from build123d import *

# Parameters (mm, degrees)
F0_W     = 30.0482
F0_H     = 30.0482
F1_DEPTH = 28.3972
F2_W     = 26.543
F2_H     = 26.543
F3_DEPTH = 27.1272
F4_R     = 0.508


with BuildPart() as f1:
    # F0 (on Front) → F1 (new body)
    with BuildSketch(Plane.XZ):
        with Locations((1.779277, -2.752393)):
            Rectangle(F0_W, F0_H)
    extrude(amount=F1_DEPTH)

    # F2 (on face) → F3 (cut)
    with BuildSketch(Plane.XZ.offset(28.3972)):
        with Locations((1.804677, -2.777793)):
            Rectangle(F2_W, F2_H)
    extrude(amount=-F3_DEPTH, mode=Mode.SUBTRACT)

    # F4
    f4_edges = [f1.edges().sort_by_distance(p)[0] for p in [
        (-13.244823, -14.1986, 12.271707),
        (-13.244823, -14.1986, -17.776493),
        (16.803377, -14.1986, 12.271707),
        (16.803377, -14.1986, -17.776493),
    ]]
    fillet(f4_edges, radius=F4_R)


solid = f1.part
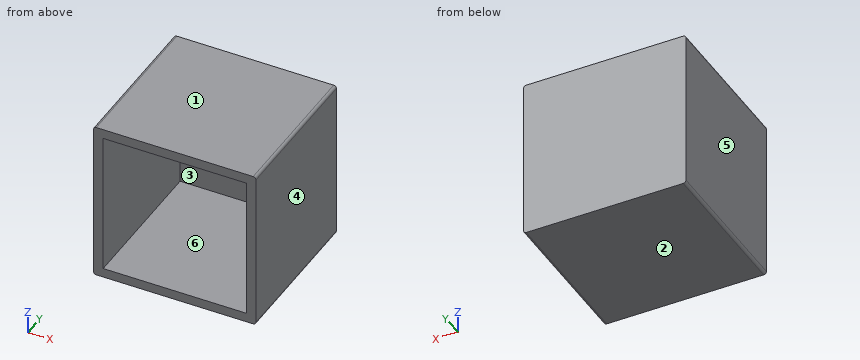
Read the model definition and answer for the solid it produces. Units are mm, in the model's axes. Face numbers are marked on the shaded views. A direction names the side the tool comes from. Coordinates: 2 decimals unless noted, no trailing zeros. Loops run counter-clockwise (first coordinate to the right, second up) from the corner with the lowest first, then second, coordinate; pieces in that order, holes last. Notation, with made-up numbers: (-9.5, 75.5) - (31.5, 75.5) arc R34 ccw to (31.5, 113.5) - close; hole circle Ø9 at (50, 8.25). An arc over 180 degrees is marked (long way). Answer in a Markdown table with one row per item.
Q1. For the marked faces 5 and 6, determine the directions among +Z, -Z, +X, -X, +Y, -Y from which every point of the face is accessible in a straight line to the end or side of a thin tool.
Here are the results:
| item | result |
|---|---|
| face 5 | +Z, -Z, -X, +Y, -Y |
| face 6 | -Y |
Q2. Find section C-C on z = 6.5. Write down the section's boundary in (x, y), plus the area to 3 significant figures.
Here are the results:
| item | result |
|---|---|
| outline | (-13.24, -28.4) - (-11.47, -28.4) - (-11.47, -1.27) - (15.08, -1.27) - (15.08, -28.4) - (16.8, -28.4) - (16.8, 0) - (-13.24, 0) - close |
| area | 133 mm^2 |
Q3. The mould has two halves that part along Z. Classify the marked faces 1, 2, 3 and 4: pulls with the +Z half, pulls with the -Z half, needs draft (parallel to the pull), parting line crosses it, or undercut.
Here are the results:
| item | result |
|---|---|
| face 1 | pulls with the +Z half |
| face 2 | pulls with the -Z half |
| face 3 | undercut |
| face 4 | needs draft |
Q4. Find section B-B on x = 2.5. Write down the section's boundary in (y, z).
Here are the results:
| item | result |
|---|---|
| outline | (-28.4, -17.78) - (0, -17.78) - (0, 12.27) - (-28.4, 12.27) - (-28.4, 10.49) - (-1.27, 10.49) - (-1.27, -16.05) - (-28.4, -16.05) - close |
Q5. Given P1, Ø1.5, axis at x = -8, z = -8.5, coming from the -Y side, flat-ended and moving along its own axis, determine where the tip first touches the part or whether it passes through.
Here are the results:
| item | result |
|---|---|
| P1 | stops at y = -1.27 |
Q6. Straight lines are drawn through the part: line 1 along X through (y, z) = (-10.5, -2.5); line 2 along Z through (x, y) = (-8.5, -24); line 3 along Y through (x, z) = (3, -9). For each, find the intervals that lie inside material, in ascending order. Write a range as [from, to].
Here are the results:
| item | result |
|---|---|
| line 1 | x = [-13.24, -11.47], [15.08, 16.8] |
| line 2 | z = [-17.78, -16.05], [10.49, 12.27] |
| line 3 | y = [-1.27, 0] |
Q7. Find section A-A on y = -2. Write down the section's boundary in (x, z), plus the area to 3 significant figures.
Here are the results:
| item | result |
|---|---|
| outline | (-13.24, -17.27) arc R0.51 ccw to (-12.74, -17.78) - (16.3, -17.78) arc R0.51 ccw to (16.8, -17.27) - (16.8, 11.76) arc R0.51 ccw to (16.3, 12.27) - (-12.74, 12.27) arc R0.51 ccw to (-13.24, 11.76) - close; hole (-11.47, -16.05) - (15.08, -16.05) - (15.08, 10.49) - (-11.47, 10.49) - close |
| area | 198 mm^2 |
